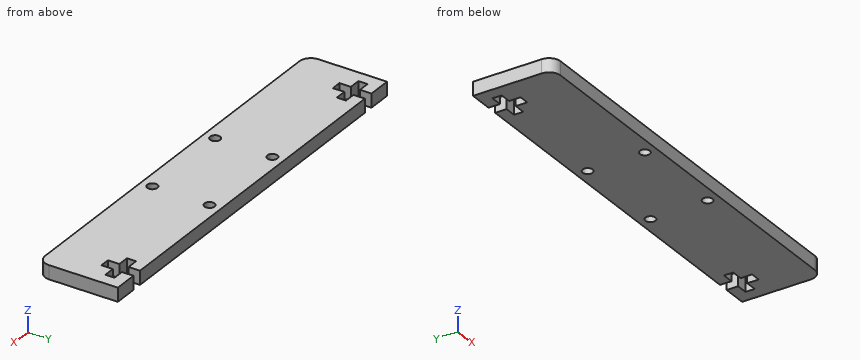
from build123d import *

# Parameters (mm, degrees)
SKETCH1_R           = 1.1
BOSS_EXTRUDE1_DEPTH = 3
FILLET1_R           = 2.5


with BuildPart() as part:
    # Sketch1 → Boss-Extrude1 (new body)
    with BuildSketch(Plane.XY):
        Polygon((-45, -8.75), (45, -8.75), (45, 8.75), (39.8, 8.75), (39.8, 6.25), (42.3, 6.25), (42.3, 4.25), (39.8, 4.25), (39.8, 1.75), (37.6, 1.75), (37.6, 4.25), (35.1, 4.25), (35.1, 6.25), (37.6, 6.25), (37.6, 8.75), (-37.6, 8.75), (-37.6, 6.25), (-35.1, 6.25), (-35.1, 4.25), (-37.6, 4.25), (-37.6, 1.75), (-39.8, 1.75), (-39.8, 4.25), (-42.3, 4.25), (-42.3, 6.25), (-39.8, 6.25), (-39.8, 8.75), (-45, 8.75), align=None)
        with Locations((-10.5, 6.25)):
            Circle(SKETCH1_R, mode=Mode.SUBTRACT)
        with Locations(Location((-10.5, -6.25, 0), (0, 0, 180))):
            Circle(SKETCH1_R, mode=Mode.SUBTRACT)
        with Locations((10.5, -6.25)):
            Circle(SKETCH1_R, mode=Mode.SUBTRACT)
        with Locations(Location((10.5, 6.25, 0), (0, 0, 180))):
            Circle(SKETCH1_R, mode=Mode.SUBTRACT)
    extrude(amount=BOSS_EXTRUDE1_DEPTH)

    # Fillet1
    fillet1_edges = [part.edges().sort_by_distance(p)[0] for p in [
        (45, -8.75, 1.5),
        (-45, -8.75, 1.5),
    ]]
    fillet(fillet1_edges, radius=FILLET1_R)


solid = part.part
Could you check a few things on this model? Use its own coordinates, in mm. Give positions to 0.01 mm unless a question says otherwise; leave off trailing zeros. Loops run counter-clockwise (first coordinate to the right, second up) from the corner with the lowest first, then second, coordinate; pieces in that order, holes last. Notation, with made-up numbers: (16.25, -10) -> (72.25, -10) arc R35 cw to (72.25, 23) -> close; hole circle Ø8 at (72.25, -22.5). An arc over 180 degrees is marked (long way). Answer as CSV lines item,"result". Start each with the question number.
(1) I'm going to push a flat-ended pin straight in: pin 1 Ø1.1 at (x, z) = (-38.5, 2) entering from +Y. Where does the tip first touch, or does it pass through?
(2) If we section it at B-B on z = 0.8: Count the separate pieces of the cut face and the enclosed holes in it, then the cut area to 3 significant figures.
(3) I need wall thicknesses on probe 1 along Y at (x, z) = (10.5, 2.15); probe 2 along X at (y, z) = (3.5, 0.55); probe 3 along X at (y, z) = (6, 1.5). Which ranges of each line are inside material? Lowest first, please.
(4) If we section it at A-A on x = 10.5: Write out the boundary of the cut face in (y, z).
Computed:
1,pin 1,"stops at y = 1.75"
2,separate pieces,"1"
2,enclosed holes,"4"
2,area,"1,510 mm2"
3,probe 1,"y = -8.75 to -7.35, -5.15 to 5.15, 7.35 to 8.75"
3,probe 2,"x = -45 to -39.8, -37.6 to 37.6, 39.8 to 45"
3,probe 3,"x = -45 to -42.3, -35.1 to -11.57, -9.43 to 9.43, 11.57 to 35.1, 42.3 to 45"
4,outline,"(-8.75, 0) -> (-7.35, 0) -> (-7.35, 3) -> (-8.75, 3) -> close; (-5.15, 0) -> (5.15, 0) -> (5.15, 3) -> (-5.15, 3) -> close; (7.35, 0) -> (8.75, 0) -> (8.75, 3) -> (7.35, 3) -> close"
